Here's how the part is built. I have some questions about the finished solid (model axes, mm). Face numbers are marked on the shaded views. A direction names the side the tool comes from. Round coordinates to 2 decimals unless told otherwise and drop trailing zeros. Write each loop counter-clockwise with the first axis right and the second up, starting at its lowest first coordinate (ties: lowest second). Pieces come first, ordered by that corner, then holes. Notation, with made-up numbers: (8, 0) - (21, 0) arc R29 ccw to (21, 25) - close; hole circle Ø8 at (-14, 40). An arc over 180 degrees is marked (long way). One line per question, with ' | ' between items. Start each with the question number.
(1) Imagine slicing it at B-B (x = 13). Write out the boundary of the cut face in (y, z), plus the area to 3 significant figures.
(2) If I drill on L1, parallel to X at y = 2.75, z = 7; L2, parallel to X at y = 10.7, z = 0; L3, parallel to Y at x = 2, z = -3, over which ranges is the centre line in solid material (lowest first)?
(3) Imagine slicing it at A-A (y = 0). Write out the boundary of the cut face in (x, z).
(4) Thinking about a two-plate mould opening in Y: for the marked faces 1, 2 and 3, which applies, pulls with the +Y half, pulls with the -Y half, needs draft (parallel to the pull), parting line crosses it, or undercut?
(5) Imagine slicing it at C-C (x = 17.25). Write out the boundary of the cut face in (y, z), plus the area to 3 significant figures.
(6) For the marked faces 4, 5 and 6, which set-ups out of +Z, -Z, +X, -X, +Y, -Y let a thin tool reach every point of the face, with its end or its side?
(7) Will these pins go through, and if not, where does the flat tip stop? pin 1 (4 mm diameter, centred on x = 16.5, z = -8.5, fed in from -Y); pin 2 (10 mm diameter, centred on y = 2, z = 1, fed in from +X); pin 3 (3.5 mm diameter, centred on x = 15.8, z = 0, fed in from +Y); pin 4 (2.5 mm diameter, centred on y = -6.3, z = 0, fed in from -X).
(8) Imagine slicing it at D-D (x = 2.75). Write out the boundary of the cut face in (y, z).
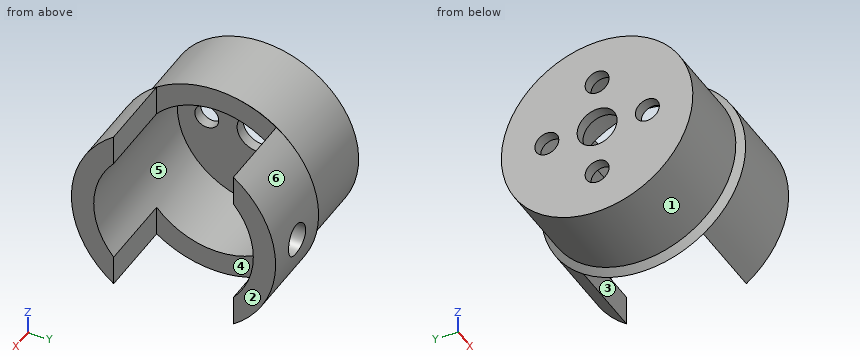
from build123d import *

# Parameters (mm, degrees)
ENL_V_MAT_EXTRU_1_REACH      = 29.571
ESQUISSE2_R                  = 2.5
ESQUISSE2_R_2                = 1.5
ENL_V_MAT_EXTRU_2_DEPTH      = 28.571390703
ENL_V_MAT_EXTRU_2_DEPTH_BACK = 28.571390703
ESQUISSE4_W                  = 15
ESQUISSE4_H                  = 10
ESQUISSE5_R                  = 2
ENL_V_MAT_EXTRU_3_DEPTH      = 10


with BuildPart() as part:
    # Esquisse1 → Révolution1 (revolve)
    with BuildSketch(Plane.XY, mode=Mode.PRIVATE) as r_volution1_sk:
        Polygon((0, 12), (10, 12), (10.798508391, 12.798508391), (20.798508391, 12.798508391), (20.798508391, 10.798508391), (20.798508391, 10), (12.242640687, 10), (1.360795334, 10), (1.360795334, 0), (0, 0), (0, 10), align=None)
    revolve(r_volution1_sk.sketch.rotate(Axis((0, 0, 0), (1, 0, 0)), 90), axis=Axis((0, 0, 0), (1, 0, 0)))

    # Esquisse2 → Enlèv. mat.-Extru.1 (cut, up to next)
    with BuildSketch(Plane.ZY, mode=Mode.PRIVATE) as enl_v_mat_extru_1_sk1:
        Circle(ESQUISSE2_R)
    enl_v_mat_extru_1_tool1 = extrude(enl_v_mat_extru_1_sk1.sketch, amount=-ENL_V_MAT_EXTRU_1_REACH, mode=Mode.PRIVATE) & part.part
    # Esquisse2 → Enlèv. mat.-Extru.1 (cut, up to next)
    with BuildSketch(Plane.ZY, mode=Mode.PRIVATE) as enl_v_mat_extru_1_sk2:
        with Locations((0, 6.3)):
            Circle(ESQUISSE2_R_2)
    enl_v_mat_extru_1_tool2 = extrude(enl_v_mat_extru_1_sk2.sketch, amount=-ENL_V_MAT_EXTRU_1_REACH, mode=Mode.PRIVATE) & part.part
    # Esquisse2 → Enlèv. mat.-Extru.1 (cut, up to next)
    with BuildSketch(Plane.ZY, mode=Mode.PRIVATE) as enl_v_mat_extru_1_sk3:
        with Locations((6.3, 0)):
            Circle(ESQUISSE2_R_2)
    enl_v_mat_extru_1_tool3 = extrude(enl_v_mat_extru_1_sk3.sketch, amount=-ENL_V_MAT_EXTRU_1_REACH, mode=Mode.PRIVATE) & part.part
    # Esquisse2 → Enlèv. mat.-Extru.1 (cut, up to next)
    with BuildSketch(Plane.ZY, mode=Mode.PRIVATE) as enl_v_mat_extru_1_sk4:
        with Locations((0, -6.3)):
            Circle(ESQUISSE2_R_2)
    enl_v_mat_extru_1_tool4 = extrude(enl_v_mat_extru_1_sk4.sketch, amount=-ENL_V_MAT_EXTRU_1_REACH, mode=Mode.PRIVATE) & part.part
    # Esquisse2 → Enlèv. mat.-Extru.1 (cut, up to next)
    with BuildSketch(Plane.ZY, mode=Mode.PRIVATE) as enl_v_mat_extru_1_sk5:
        with Locations((-6.3, 0)):
            Circle(ESQUISSE2_R_2)
    enl_v_mat_extru_1_tool5 = extrude(enl_v_mat_extru_1_sk5.sketch, amount=-ENL_V_MAT_EXTRU_1_REACH, mode=Mode.PRIVATE) & part.part
    add(enl_v_mat_extru_1_tool1.solids().sort_by_distance((0, 0, 0))[0], mode=Mode.SUBTRACT)
    add(enl_v_mat_extru_1_tool2.solids().sort_by_distance((0, 6.3, 0))[0], mode=Mode.SUBTRACT)
    add(enl_v_mat_extru_1_tool3.solids().sort_by_distance((0, 0, 6.3))[0], mode=Mode.SUBTRACT)
    add(enl_v_mat_extru_1_tool4.solids().sort_by_distance((0, -6.3, 0))[0], mode=Mode.SUBTRACT)
    add(enl_v_mat_extru_1_tool5.solids().sort_by_distance((0, 0, -6.3))[0], mode=Mode.SUBTRACT)

    # Esquisse4 → Enlèv. mat.-Extru.2 (cut, two sides: drawn at the far end of the back side and taken through both)
    with BuildSketch(Plane.YX.offset(-ENL_V_MAT_EXTRU_2_DEPTH_BACK)):
        with Locations((0.001491609, 15.798508391)):
            Rectangle(ESQUISSE4_W, ESQUISSE4_H)
    extrude(amount=ENL_V_MAT_EXTRU_2_DEPTH + ENL_V_MAT_EXTRU_2_DEPTH_BACK, mode=Mode.SUBTRACT)

    # Esquisse5 → Enlèv. mat.-Extru.3 (cut)
    with BuildSketch(Plane(origin=(0, 12.798508391, 0), x_dir=(1, 0, 0), z_dir=(0, 1, 0))):
        with Locations(Location((15.798508391, 0, 0), (0, 0, 270))):
            Circle(ESQUISSE5_R)
    extrude(amount=-ENL_V_MAT_EXTRU_3_DEPTH, mode=Mode.SUBTRACT)


solid = part.part
Check sheet entries:
1) outline: (-7.5, -10.37) - (-7.5, -6.62) arc R10 cw to (-7.5, 6.62) - (-7.5, 10.37) arc R12.8 ccw to start; (7.5, -10.37) arc R12.8 ccw to (7.5, 10.37) - (7.5, 6.61) arc R10 cw to (7.5, -6.61) - close | area: 109 mm^2
2) L1: 0 to 1.36 | L2: 0 to 13.8, 17.8 to 20.8 | L3: -11.62 to -9.54, 9.54 to 11.62
3) outline: (0, -12) - (10, -12) - (10.8, -12.8) - (10.8, -10) - (1.36, -10) - (1.36, -7.8) - (0, -7.8) - close; (0, -4.8) - (1.36, -4.8) - (1.36, -2.5) - (0, -2.5) - close; (0, 2.5) - (1.36, 2.5) - (1.36, 4.8) - (0, 4.8) - close; (0, 7.8) - (1.36, 7.8) - (1.36, 10) - (10.8, 10) - (10.8, 12.8) - (10, 12) - (0, 12) - close
4) face 1: parting line crosses it | face 2: needs draft | face 3: undercut
5) outline: (-7.5, -10.37) - (-7.5, -6.62) arc R10 cw to (-7.5, 6.62) - (-7.5, 10.37) arc R12.8 ccw to start; (7.5, -10.37) arc R12.8 ccw to (12.72, -1.38) - (9.9, -1.38) arc R10 cw to (7.5, -6.61) - close; (7.5, 6.61) arc R10 cw to (9.9, 1.38) - (12.72, 1.38) arc R12.8 ccw to (7.5, 10.37) - close | area: 101 mm^2
6) face 4: +Z, -Z, +X | face 5: +X | face 6: +X, -X, +Y
7) pin 1: y = -11.03 | pin 2: x = 1.36 | pin 3: y = -9.85 | pin 4: through
8) outline: circle Ø24 at (0, 0); hole circle Ø20 at (0, 0)
